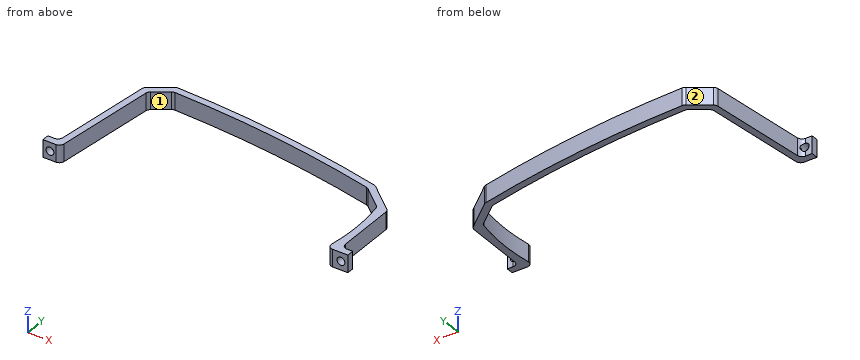
from build123d import *

# Parameters (mm, degrees)
BOSS_EXTRU_1_DEPTH           = 10
ESQUISSE2_W                  = 10
ESQUISSE2_H                  = 4
BOSS_EXTRU_2_DEPTH           = 10
ENL_V_MAT_EXTRU_1_DEPTH      = 180.426169252
ENL_V_MAT_EXTRU_1_DEPTH_BACK = 180.426169252
ESQUISSE3_R                  = 2.25
CONG_1_START                 = -1
CONG_1_DEPTH                 = 12
CONG_1_START_2               = 7.2500001
CONG_1_2_DEPTH               = 2.7499999
CONG_1_3_DEPTH               = 2.749998557
CONG_1_START_3               = 1.0274
CONG_1_4_DEPTH               = 7.9164
CONG_1_START_4               = 2.749998557
CONG_1_5_DEPTH               = 4.500001543
CONG_1_START_5               = 4
CONG_1_6_OUTLINE_R           = 2.25
CONG_1_6_DEPTH               = 2.645361331


with BuildPart() as part:
    # Esquisse1 → Boss.-Extru.1 (new body)
    with BuildSketch(Plane.XY):
        with BuildLine():
            Line((0, 0), (7.380952381, 62))
            Line((7.380952381, 62), (17.380952381, 69))
            ThreePointArc((17.380952381, 69), (79.097781351, 63.974797541), (140.038518603, 53))
            Line((140.038518603, 53), (153, 42))
            ThreePointArc((153, 42), (155, 21), (153, 0))
            Line((153, 0), (159, 0))
            Line((159, 0), (159, 42.15430335))
            Line((159, 42.15430335), (156.65156229, 44.147348282))
            Line((156.65156229, 44.147348282), (141.886380642, 56.678091733))
            ThreePointArc((141.886380642, 56.678091733), (79.436142512, 67.964522606), (16.177522156, 73.040221089))
            Line((16.177522156, 73.040221089), (3.620610131, 64.250382671))
            Line((3.620610131, 64.250382671), (-3.971953097, 0.472851559))
            Line((-3.971953097, 0.472851559), (-3.971953097, 0))
            Line((-3.971953097, 0), (0, 0))
        make_face()
    extrude(amount=BOSS_EXTRU_1_DEPTH)

    # Esquisse2 → Boss.-Extru.2 (add)
    with BuildSketch(Plane.XY.offset(10)):
        with Locations((-5, 2)):
            Rectangle(ESQUISSE2_W, ESQUISSE2_H)
        Polygon((155.309401077, 4), (153, 0), (165.309401077, 0), (165.309401077, 4), align=None)
    extrude(amount=-BOSS_EXTRU_2_DEPTH)

    # Esquisse3 → Enlèv. mat.-Extru.1 (cut, two sides: drawn at the far end of the back side and taken through both)
    with BuildSketch(Plane(origin=(0, 4, 0), x_dir=(1, 0, 0), z_dir=(0, 1, 0)).offset(-ENL_V_MAT_EXTRU_1_DEPTH_BACK)):
        with Locations(Location((-6, -5, 0), (0, 0, 180))):
            Circle(ESQUISSE3_R)
        with Locations(Location((161.309401077, -5, 0), (0, 0, 180))):
            Circle(ESQUISSE3_R)
    extrude(amount=ENL_V_MAT_EXTRU_1_DEPTH + ENL_V_MAT_EXTRU_1_DEPTH_BACK, mode=Mode.SUBTRACT)

    # Congé1: read off the stored shape, not the designer's step
    # Congé1 outline → Congé1 (cut)
    with BuildSketch(Plane.XY.offset(CONG_1_START)):
        with BuildLine():
            Line((16.177522156, 73.040221089), (15.360062357, 72.46799923))
            ThreePointArc((15.360062357, 72.46799923), (16.22479158, 72.885690349), (17.177199346, 73.00874297))
            ThreePointArc((17.177199346, 73.00874297), (16.677366871, 73.02467639), (16.177522156, 73.040221089))
        make_face()
        with BuildLine():
            ThreePointArc((3.461901996, 62.917234337), (3.866631155, 64.103151006), (4.720479785, 65.020291429))
            Line((4.720479785, 65.020291429), (3.620610131, 64.250382671))
            Line((3.620610131, 64.250382671), (3.461901996, 62.917234337))
        make_face()
        with BuildLine():
            Line((159, 42.15430335), (157.941176471, 43.052893447))
            ThreePointArc((157.941176471, 43.052893447), (158.722455639, 42.025825276), (159, 40.7655732))
            Line((159, 40.7655732), (159, 42.15430335))
        make_face()
        with BuildLine():
            ThreePointArc((141.886380642, 56.678091733), (141.530964579, 56.760515154), (141.175501808, 56.842736905))
            ThreePointArc((141.175501808, 56.842736905), (141.846525936, 56.600679011), (142.441431075, 56.207037956))
            Line((142.441431075, 56.207037956), (141.886380642, 56.678091733))
        make_face()
        with BuildLine():
            Line((0, 0), (0.314923968, 2.645361331))
            ThreePointArc((0.314923968, 2.645361331), (-0.672046378, 0.756797378), (-2.664040855, 0))
            Line((-2.664040855, 0), (0, 0))
        make_face()
        with BuildLine():
            ThreePointArc((156.573147005, 0), (154.290829859, 1.052943646), (153.610613604, 3.472647702))
            ThreePointArc((153.610613604, 3.472647702), (153.319065292, 1.733904625), (153, 0))
            Line((153, 0), (156.573147005, 0))
        make_face()
    extrude(amount=CONG_1_DEPTH, mode=Mode.SUBTRACT)

    # Cong_1 2 outline → Cong_1 2 (add)
    with BuildSketch(Plane.XY.offset(CONG_1_START_2)):
        with BuildLine():
            Line((-3.552054473, 4), (-3.237130505, 6.645361331))
            ThreePointArc((-3.237130505, 6.645361331), (-4.224100851, 4.756797378), (-6.216095328, 4))
            Line((-6.216095328, 4), (-3.552054473, 4))
        make_face()
        with BuildLine():
            ThreePointArc((162, 4), (159.878679656, 4.878679656), (159, 7))
            Line((159, 7), (159, 4))
            Line((159, 4), (162, 4))
        make_face()
        with BuildLine():
            Line((153, 42), (152.188329288, 42.688839304))
            ThreePointArc((152.188329288, 42.688839304), (152.845168439, 41.901623997), (153.198575067, 40.939205498))
            ThreePointArc((153.198575067, 40.939205498), (153.100573868, 41.469843544), (153, 42))
        make_face()
        with BuildLine():
            ThreePointArc((7.222244246, 60.666851666), (7.626973405, 61.852768335), (8.480822035, 62.769908758))
            Line((8.480822035, 62.769908758), (7.380952381, 62))
            Line((7.380952381, 62), (7.222244246, 60.666851666))
        make_face()
        with BuildLine():
            ThreePointArc((16.560647408, 68.425786519), (17.428384152, 68.844370904), (18.384055662, 68.96632134))
            ThreePointArc((18.384055662, 68.96632134), (17.882510633, 68.983357604), (17.380952381, 69))
            Line((17.380952381, 69), (16.560647408, 68.425786519))
        make_face()
        with BuildLine():
            ThreePointArc((139.325020621, 53.164109281), (139.998459684, 52.922050789), (140.595410438, 52.527383484))
            Line((140.595410438, 52.527383484), (140.038518603, 53))
            ThreePointArc((140.038518603, 53), (139.681793114, 53.08215682), (139.325020621, 53.164109281))
        make_face()
    extrude(amount=CONG_1_2_DEPTH)

    # Cong_1 3 outline → Cong_1 3 (add)
    with BuildSketch(Plane.XY):
        with BuildLine():
            Line((-3.552054473, 4), (-3.237130505, 6.645361331))
            ThreePointArc((-3.237130505, 6.645361331), (-4.224100851, 4.756797378), (-6.216095328, 4))
            Line((-6.216095328, 4), (-3.552054473, 4))
        make_face()
        with BuildLine():
            ThreePointArc((162, 4), (159.878679656, 4.878679656), (159, 7))
            Line((159, 7), (159, 4))
            Line((159, 4), (162, 4))
        make_face()
        with BuildLine():
            Line((153, 42), (152.188329288, 42.688839304))
            ThreePointArc((152.188329288, 42.688839304), (152.845168439, 41.901623997), (153.198575067, 40.939205498))
            ThreePointArc((153.198575067, 40.939205498), (153.100573868, 41.469843544), (153, 42))
        make_face()
        with BuildLine():
            ThreePointArc((7.222244246, 60.666851666), (7.626973405, 61.852768335), (8.480822035, 62.769908758))
            Line((8.480822035, 62.769908758), (7.380952381, 62))
            Line((7.380952381, 62), (7.222244246, 60.666851666))
        make_face()
        with BuildLine():
            ThreePointArc((16.560647408, 68.425786519), (17.428384152, 68.844370904), (18.384055662, 68.96632134))
            ThreePointArc((18.384055662, 68.96632134), (17.882510633, 68.983357604), (17.380952381, 69))
            Line((17.380952381, 69), (16.560647408, 68.425786519))
        make_face()
        with BuildLine():
            ThreePointArc((139.325020621, 53.164109281), (139.998459684, 52.922050789), (140.595410438, 52.527383484))
            Line((140.595410438, 52.527383484), (140.038518603, 53))
            ThreePointArc((140.038518603, 53), (139.681793114, 53.08215682), (139.325020621, 53.164109281))
        make_face()
    extrude(amount=CONG_1_3_DEPTH)

    # Cong_1 4 outline → Cong_1 4 (add)
    with BuildSketch(Plane.XY.offset(CONG_1_START_3)):
        with BuildLine():
            Line((153, 42), (152.188329288, 42.688839304))
            ThreePointArc((152.188329288, 42.688839304), (152.845168439, 41.901623997), (153.198575067, 40.939205498))
            ThreePointArc((153.198575067, 40.939205498), (153.100573868, 41.469843544), (153, 42))
        make_face()
        with BuildLine():
            ThreePointArc((7.222244246, 60.666851666), (7.626973405, 61.852768335), (8.480822035, 62.769908758))
            Line((8.480822035, 62.769908758), (7.380952381, 62))
            Line((7.380952381, 62), (7.222244246, 60.666851666))
        make_face()
        with BuildLine():
            ThreePointArc((16.560647408, 68.425786519), (17.428384152, 68.844370904), (18.384055662, 68.96632134))
            ThreePointArc((18.384055662, 68.96632134), (17.882510633, 68.983357604), (17.380952381, 69))
            Line((17.380952381, 69), (16.560647408, 68.425786519))
        make_face()
        with BuildLine():
            ThreePointArc((139.325020621, 53.164109281), (139.998459684, 52.922050789), (140.595410438, 52.527383484))
            Line((140.595410438, 52.527383484), (140.038518603, 53))
            ThreePointArc((140.038518603, 53), (139.681793114, 53.08215682), (139.325020621, 53.164109281))
        make_face()
    extrude(amount=CONG_1_4_DEPTH)

    # Cong_1 5 outline → Cong_1 5 (add)
    with BuildSketch(Plane.XY.offset(CONG_1_START_4)):
        with BuildLine():
            Line((159, 4), (162, 4))
            ThreePointArc((162, 4), (159.878679656, 4.878679656), (159, 7))
            Line((159, 7), (159, 4))
        make_face()
        with BuildLine():
            ThreePointArc((-3.237130505, 6.645361331), (-4.224100851, 4.756797378), (-6.216095328, 4))
            Line((-6.216095328, 4), (-3.552054473, 4))
            Line((-3.552054473, 4), (-3.237130505, 6.645361331))
        make_face()
    extrude(amount=CONG_1_5_DEPTH)

    # Cong_1 6 outline → Cong_1 6 (cut)
    with BuildSketch(Plane(origin=(0, 0, 0), x_dir=(1, 0, 0), z_dir=(0, 1, 0)).offset(CONG_1_START_5)):
        with Locations((161.309401077, -5)):
            Circle(CONG_1_6_OUTLINE_R)
        with Locations((-6, -5)):
            Circle(CONG_1_6_OUTLINE_R)
    extrude(amount=CONG_1_6_DEPTH, mode=Mode.SUBTRACT)


solid = part.part
The model under review builds one solid part; all positions refer to its coordinate system, in mm. Face numbers are marked on the shaded views. A direction names the side the tool comes from. Coordinates: 2 decimals unless noted, no trailing zeros. Order: outer loops, then holes, each group sorted by start corner. A loop starts at its lowest first (then second) coordinate and runs counter-clockwise, first axis right, second up. Notation, with made-up numbers: (-27, 37) -> (-6, 37) arc R22 ccw to (-6, 61) -> close; hole circle Ø4 at (52.5, 50). An arc over 180 degrees is marked (long way). Answer in a Markdown table with one row per item.
(1) Wall thickness on line 1 along X through (y, z) = (2.7, 5); line 2 along Z through (x, y) = (-6, 2.7); line 3 along X through (y, z) = (3, 5): over which ranges is each line inside the solid? List them lowest first.
Answers:
| item | result |
|---|---|
| line 1 | -10 to -8.25, -3.75 to 0.32, 153.59 to 159.06, 163.56 to 165.31 |
| line 2 | 0 to 2.75, 7.25 to 10 |
| line 3 | -10 to -8.25, -3.75 to 0.36, 153.57 to 159.06, 163.56 to 165.31 |
(2) Consider section A-A (y = 29.5). Write out the cut boundary in (x, z).
Answers:
| item | result |
|---|---|
| outline | (-0.52, 0) -> (3.51, 0) -> (3.51, 10) -> (-0.52, 10) -> close; (154.67, 0) -> (159, 0) -> (159, 10) -> (154.67, 10) -> close |
(3) Consider section D-D (x = 64.5). Write out the cut boundary in (y, z).
Answers:
| item | result |
|---|---|
| outline | (65.71, 0) -> (69.73, 0) -> (69.73, 10) -> (65.71, 10) -> close |
(4) Consider section C-C (x = 94). Write out the cut boundary in (y, z), plus the area to 3 significant figures.
Answers:
| item | result |
|---|---|
| outline | (61.85, 0) -> (65.9, 0) -> (65.9, 10) -> (61.85, 10) -> close |
| area | 40.5 mm² |
(5) Consider section B-B (y = 20). Write out the cut boundary in (x, z), plus the area to 3 significant figures.
Answers:
| item | result |
|---|---|
| outline | (-1.65, 0) -> (2.38, 0) -> (2.38, 10) -> (-1.65, 10) -> close; (155, 0) -> (159, 0) -> (159, 10) -> (155, 10) -> close |
| area | 80.3 mm² |
(6) Insertion check: pin 1 (6 mm diameter, centred on x = 29.5, z = 3, fed in from +Y); pin 2 (6 mm diameter, centred on x = 115, z = 5.5, fed in from -Y); pin 3 (3 mm diameter, centred on x = -8, z = 7.5, fed in from +Y). Each pin has a flat end and moves straight along its axis. Give the tip position at first contact, or say it passes through.
Answers:
| item | result |
|---|---|
| pin 1 | y = 72.64 |
| pin 2 | y = 57.67 |
| pin 3 | y = 4 |
(7) Machinability: for the marked faces 1 and 2, which of the approach directions +Z, -Z, +X, -X, +Y, -Y give a long, thin tool a straight path to every point of the face, cutting with its end or side? Answer none if there is none.
Answers:
| item | result |
|---|---|
| face 1 | +Z, -Z, -Y |
| face 2 | +Z, -Z, -X, +Y |
